from build123d import *

# Parameters (mm, degrees)
SKETCH_1_W          = 78
SKETCH_1_H          = 66
EXTRUDE_1_DEPTH     = 34
SKETCH_1_3_W        = 30
SKETCH_1_3_H        = 66
EXTRUDE_2_DEPTH     = 70
SKETCH_2_R          = 18
CUT_EXTRUDE_1_DEPTH = 23
SKETCH_3_R          = 24.5
CUT_EXTRUDE_2_DEPTH = 70
CUT_EXTRUDE_3_REACH = 134.865


with BuildPart() as part:
    # Sketch 1 → Extrude 1 (new body)
    with BuildSketch(Plane(origin=(0, 0, 0), x_dir=(1, 0, 0), z_dir=(0, 1, 0))):
        with Locations((-15, 0)):
            Rectangle(SKETCH_1_W, SKETCH_1_H)
    extrude(amount=EXTRUDE_1_DEPTH)

    # Sketch 1_3 → Extrude 2 (add)
    with BuildSketch(Plane(origin=(0, 0, 0), x_dir=(1, 0, 0), z_dir=(0, 1, 0))):
        with Locations((39, 0)):
            Rectangle(SKETCH_1_3_W, SKETCH_1_3_H)
    extrude(amount=EXTRUDE_2_DEPTH)

    # Sketch 2 → Cut-Extrude 1 (cut)
    with BuildSketch(Plane(origin=(0, 34, 0), x_dir=(1, 0, 0), z_dir=(0, 1, 0))):
        with Locations(Location((-15, 0, 0), (0, 0, 270))):
            Circle(SKETCH_2_R)
    extrude(amount=-CUT_EXTRUDE_1_DEPTH, mode=Mode.SUBTRACT)

    # Sketch 3 → Cut-Extrude 2 (cut)
    with BuildSketch(Plane.ZY.offset(-24)):
        with Locations((0, 70)):
            Circle(SKETCH_3_R)
    extrude(amount=-CUT_EXTRUDE_2_DEPTH, mode=Mode.SUBTRACT)

    # Sketch 4 → Cut-Extrude 3 (cut, up to next)
    with BuildSketch(Plane.ZY.offset(54), mode=Mode.PRIVATE) as cut_extrude_3_sk1:
        Polygon((21, 12), (-21, 12), (-15, 0), (15, 0), align=None)
    cut_extrude_3_tool1 = extrude(cut_extrude_3_sk1.sketch, amount=-CUT_EXTRUDE_3_REACH, mode=Mode.PRIVATE) & part.part
    add(cut_extrude_3_tool1.solids().sort_by_distance((-54, 6.333333, 0))[0], mode=Mode.SUBTRACT)


solid = part.part
CAD build for the part. Positions are in the model's coordinates, mm. A direction names the side the tool comes from. Give positions to 0.01 mm unless a question says otherwise; leave off trailing zeros. Loops run counter-clockwise (first coordinate to the right, second up) from the corner with the lowest first, then second, coordinate; pieces in that order, holes last. Notation, with made-up numbers: M -7,59.5 L 20,59.5 A22 ccw 20,79.5 Z; hole C -15.5,89.5 d3. An arc over 180 degrees is marked long. Answer in a Markdown table with one row per item. Add a question column.
Item 1: Mould opens along Z. For faces 4 (the face through (11, 19, 33)), 5 (the face through (-1, 0, 24)), 6 (the face through (-1, 6, -18)) say: +Z half, -Z half, draft (parallel to the pull), parting line (faces both ways), or undercut.
Item 2: Band-saw the part on C-C on y = 21.5. Give the cut face in (x, z), then the cut area to 3 significant figures.
Item 3: Band-saw the part on A-A on x = -15. Give the cut face in (y, z), then the cut area to 3 significant figures.
Item 4: Tool access for faces 1 (the face through (-1, 6, 18)), 2 (the face through (-25.953, 23.154, -14.284)), 3 (the face through (24, 44, 0)): list every direction of +Z, -Z, +X, -X, +Y, -Y with a clear straight run to the whole face (end or side of a thin tool).
Item 5: Probe probe 1 along X at (y, z) = (21.5, 0); probe 2 along Y at (x, z) = (-13, 18.5); probe 3 along Y at (x, z) = (-21, 19). List the from-to ranges inside material, lowest first.
Item 6: Band-saw the part on B-B on z = 0. Give the cut face in (x, y), then the cut area to 3 significant figures.
Item 7: Drop flat-ended pins along their axis: P1, Ø8, axis at x = 26, z = 7, coming from the +Y side; P2, Ø1.5, axis at x = -36.5, z = -6.5, coming from the +Y side; P3, Ø1.5, axis at y = 36.5, z = -16.5, coming from the -X side. Give the stop position or say it passes through.
Item 8: Band-saw the part on D-D on x = 42. Give the cut face in (y, z), then the cut area to 3 significant figures.
Reply:
| question | item | result |
|---|---|---|
| 1 | face 4 | +Z half |
| 1 | face 5 | draft |
| 1 | face 6 | undercut |
| 2 | outline | M -54,-33 L 54,-33 L 54,33 L -54,33 Z; hole C -15,0 d36 |
| 2 | area | 6,110 mm^2 |
| 3 | outline | M 0,-33 L 34,-33 L 34,-18 L 12,-18 L 12,-21 L 0,-15 Z; M 0,15 L 12,21 L 12,18 L 34,18 L 34,33 L 0,33 Z |
| 3 | area | 1,020 mm^2 |
| 4 | face 1 | +X, -X |
| 4 | face 2 | +Y |
| 4 | face 3 | +Z, -Z, -X, +Y |
| 5 | probe 1 | x = -54 to -33, 3 to 54 |
| 5 | probe 2 | y = 0 to 7, 12 to 34 |
| 5 | probe 3 | y = 0 to 8, 12 to 34 |
| 6 | outline | M -54,12 L -33,12 L -33,34 L -54,34 Z; M 3,12 L 54,12 L 54,45.5 L 24,45.5 L 24,34 L 3,34 Z |
| 6 | area | 1,930 mm^2 |
| 7 | P1 | stops at y = 48.11 |
| 7 | P2 | stops at y = 34 |
| 7 | P3 | stops at x = 24 |
| 8 | outline | M 0,-33 L 70,-33 L 70,-24.5 A24.5 cw 70,24.5 L 70,33 L 0,33 L 0,15 L 12,21 L 12,-21 L 0,-15 Z |
| 8 | area | 3,250 mm^2 |
